Answer from the drawing. Dimensions are ordinates in mm from the lowest x, y and z of the part. Coordinates: 2 decimals unless noted, no trailing zeros. Order: outer loops, then holes, each group sorted by start corner. A loop starts at its lowest first (then second) coordinate and runs counter-clockwise, first axis right, second up. Notation, with made-up numbers: (-9, 10.25) - (49, 10.25) arc R9 ccw to (49, 14.25) - close; hole circle Ø11 at (64, 14.25). An arc over 180 degrees is marked (long way). Use a Markdown table: item, result. Add a question column.
Item 1: Find the intervals of material crossed by line 1 along Y through (x, z) = (42.5, 2.3); line 2 along Y through (x, z) = (44, 3.85); line 3 along X through (y, z) = (52.5, 3.5), in increasing order.
Item 2: The part is cut by section C-C, the plane y = 58. Give the vertices of the cut face in (x, z).
Item 3: The part is cut by section B-B, the plane z = 3.2. Give the vertices of the cut face in (x, y).
Item 4: The part is cut by section D-D, the plane x = 72.5. Give the vertices of the cut face in (y, z).
Item 5: The part is cut by section A-A, the plane x = 42.5. Give the vertices of the cut face in (y, z).
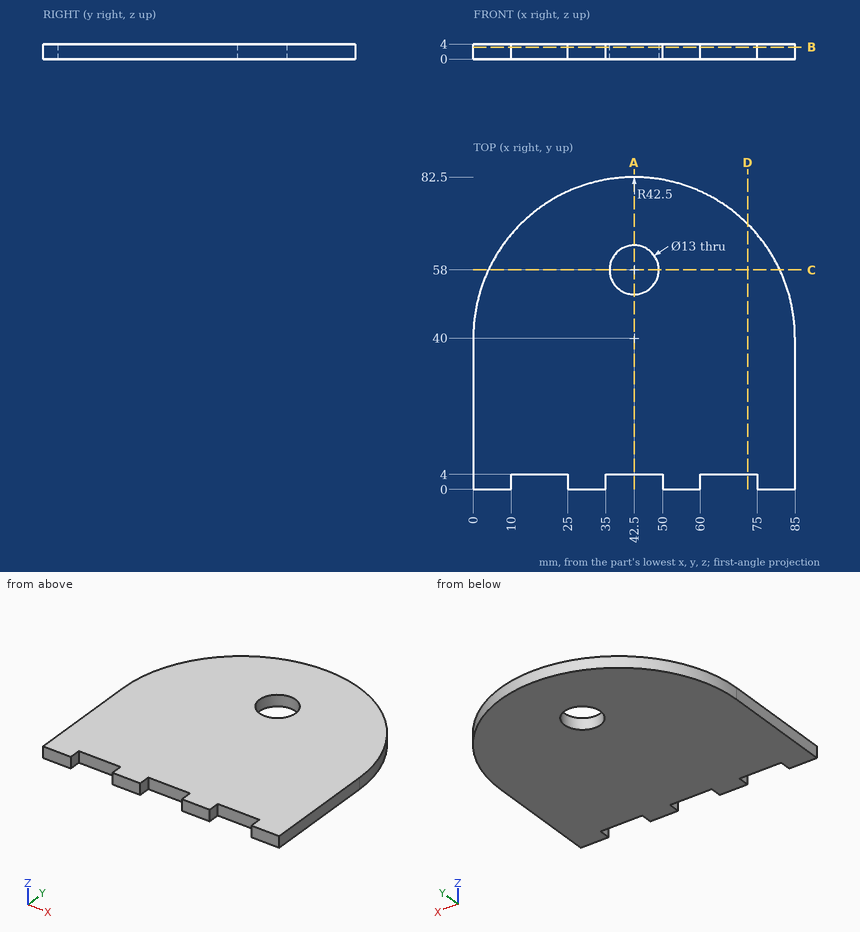
Solution:
| question | item | result |
|---|---|---|
| 1 | line 1 | y = 4 to 51.5, 64.5 to 82.5 |
| 1 | line 2 | y = 4 to 51.68, 64.32 to 82.47 |
| 1 | line 3 | x = 1.88 to 39.04, 45.96 to 83.12 |
| 2 | outline | (4, 0) - (36, 0) - (36, 4) - (4, 4) - close; (49, 0) - (81, 0) - (81, 4) - (49, 4) - close |
| 3 | outline | (0, 0) - (10, 0) - (10, 4) - (25, 4) - (25, 0) - (35, 0) - (35, 4) - (50, 4) - (50, 0) - (60, 0) - (60, 4) - (75, 4) - (75, 0) - (85, 0) - (85, 40) arc R42.5 ccw to (0, 40) - close; hole circle Ø13 at (42.5, 58) |
| 4 | outline | (4, 0) - (70.1, 0) - (70.1, 4) - (4, 4) - close |
| 5 | outline | (4, 0) - (51.5, 0) - (51.5, 4) - (4, 4) - close; (64.5, 0) - (82.5, 0) - (82.5, 4) - (64.5, 4) - close |
